Autodesk Inventor part; units mm, degrees
ref_plane "YZ Plane" through (0, 0, 0) normal (1, 0, 0) x (0, 1, 0)
ref_plane "XZ Plane" through (0, 0, 0) normal (0, 1, 0) x (-1, 0, 0)
ref_plane "XY Plane" through (0, 0, 0) normal (0, 0, 1) x (1, 0, 0)
sketch "Sketch1" plane through (0, 0, 0) normal (1, 0, 0) x (0, 1, 0)
  line L0 (-20, 32) -> (20, 32)
  line L1 (20, 32) -> (20, -32)
  line L2 (20, -32) -> (-20, -32)
  line L3 (-20, -32) -> (-20, 32)
  line L4 (-20, 32) -> (20, -32) construction
  line L5 (20, 32) -> (-20, -32) construction
  point P0 (0, 0)
  dimension "d0" = 40
  dimension "d1" = 64
extrude "Extrusion1" add sketch "Sketch1" along normal mid plane 3.175
sketch "Sketch2" plane through (1.5875, 0, 0) normal (1, 0, 0) x (0, 0, -1)
  circle A0 centre (-28, 16) radius 2
  line L0 (-32, 20) -> (-32, -20) construction
  line L1 (-32, 0) -> (32, 0) construction
  line L2 (32, -20) -> (32, 20) construction
  line L3 (32, 20) -> (-32, 20) construction
  line L4 (0, 20) -> (0, -20) construction
  circle A1 centre (28, 16) radius 2
  circle A2 centre (-28, -16) radius 2
  circle A3 centre (28, -16) radius 2
  circle A4 centre (-8, 8) radius 2
  circle A5 centre (-8, -8) radius 2
  circle A6 centre (8, -8) radius 2
  circle A7 centre (8, 8) radius 2
  circle A8 centre (0, 0) radius 7
  point P0 (0, 0)
  point P1 (0, 0)
  dimension "d4" = 4
  dimension "d5" = 28
  dimension "d6" = 16
  dimension "d7" = 4
  dimension "d8" = 8
  dimension "d9" = 8
  dimension "d12" = 360
  dimension "d14" = 14
extrude "Extrusion2" cut sketch "Sketch2" against normal through all
chamfer "Chamfer1" distance 2 angle 45 4 edges at (0, 20, 32) (0, -20, 32) (0, -20, -32) (0, 20, -32)
properties part number "TurretMotorPlate"
Can you work these out from the model? Positions are in its coordinate system, mm. Give positions to 0.01 mm unless a question says otherwise; leave off trailing zeros. Order: outer loops, then holes, each group sorted by start corner. A loop starts at its lowest first (then second) coordinate and runs counter-clockwise, first axis right, second up. Notation, with made-up numbers: M 25,4 L 32,4 A17 cw 32,34 Z; hole C 11,-8.75 d11. An arc over 180 degrees is marked long. Use one line per item in the form item = value. Start each with the question number.
Item 1: If we section it at A-A (z = 28): Write out the boundary of the cut face in (x, y).
Item 2: We'd pull the mould along Y, two halves only. Please class faces 1 (the cylindrical face through (0.022, 9.352, 9.474)), 2 (the cylindrical face through (0.022, 16.601, 26.092)), 3 (the flat face through (0, 0, -32)), 4 (the flat face through (0, 19, 31)): +Y half, -Y half, draft (parallel to the pull), parting line (faces both ways), or undercut.
Item 3: If we section it at D-D (z = 0): Write out the boundary of the cut face in (x, y).
Item 4: If I drill on line 1 along Y through (x, z) = (-0.8, -28); line 2 along Z through (x, y) = (-1.35, -9.5); line 3 along Y through (x, z) = (0.1, 26.5), over which ranges is the centre line in solid material (lowest first)?
Item 5: If we section it at C-C (x = 0.25): State how many separate pieces and enclosed holes the cut face has, then the cut area to 3 significant figures.
Item 6: If we section it at B-B (y = 0): Write out the boundary of the cut face in (x, z).
Item 7: Will this pin go through, and if not, where does the flat tip stop? pin 1 Ø3 at (y, z) = (8, 8) entering from -X.
Outcome:
q1.outline = M -1.59,-20 L 1.59,-20 L 1.59,-18 L -1.59,-18 Z; M -1.59,-14 L 1.59,-14 L 1.59,14 L -1.59,14 Z; M -1.59,18 L 1.59,18 L 1.59,20 L -1.59,20 Z
q2.face_1 = undercut
q2.face_2 = undercut
q2.face_3 = draft
q2.face_4 = +Y half
q3.outline = M -1.59,-20 L 1.59,-20 L 1.59,-7 L -1.59,-7 Z; M -1.59,7 L 1.59,7 L 1.59,20 L -1.59,20 Z
q4.line_1 = -20 to -18, -14 to 14, 18 to 20
q4.line_2 = -32 to -9.32, -6.68 to 6.68, 9.32 to 32
q4.line_3 = -20 to -17.32, -14.68 to 14.68, 17.32 to 20
q5.separate_pieces = 1
q5.enclosed_holes = 9
q5.area = 2,300 mm2
q6.outline = M -1.59,-32 L 1.59,-32 L 1.59,-7 L -1.59,-7 Z; M -1.59,7 L 1.59,7 L 1.59,32 L -1.59,32 Z
q7.pin_1 = through
